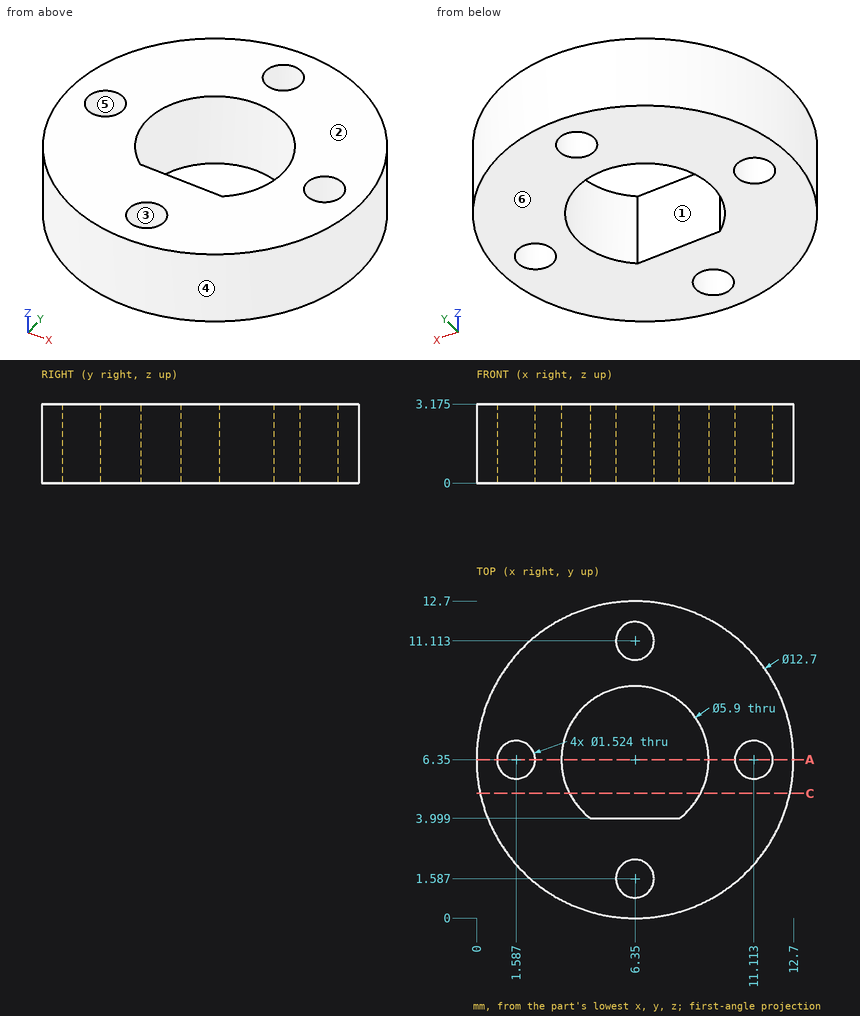
Print and shaded views of the part. All mm, measured from the part's lowest x, y and z. A direction names the side the tool comes from. Round coordinates to 2 decimals unless told otherwise and drop trailing zeros. Write each loop counter-clockwise with the first axis right and the second up, starting at its lowest first coordinate (ties: lowest second). Pieces come first, ordered by that corner, then holes. Notation, with made-up numbers: (33.25, 60) - (61.25, 60) arc R29 cw to (61.25, 92) - close; hole circle Ø1 at (26.25, 51). An arc over 180 degrees is marked (long way). Write each question's results on one line, items separated by ' | '. Start each with the question number.
Item 1: Drop flat-ended pins along their axis: P1, Ø1, axis at y = 5, z = 1, coming from the -X side; P2, Ø1.5, axis at y = 11, z = 0.5, coming from the -X side; P3, Ø1, axis at x = 1.5, z = 2.5, coming from the -Y side (1 decimal). Give the stop position or say it passes through.
Item 2: Mould opens along Y. For the marked faces 3, 4, 5 and 6 say: pulls with the +Y half, pulls with the -Y half, needs draft (parallel to the pull), parting line crosses it, or undercut.
Item 3: Saw through at A-A (y = 6.35). State how many separate pieces and enclosed holes the cut face has, and give its area (3 significant figures).
Item 4: Saw through at C-C (y = 5). Write the cut outline in (x, z) (1 decimal).
Item 5: Which spindle directions (+Z, -Z, +X, -X, +Y, -Y) get a long thin tool onto all of the face, cutting with end or side? Do the marked faces 1 and 2. Say none if no direction does.
Item 6: Wall check: L1, parallel to X at y = 7, z = 2.2 (1 decimal); L2, parallel to Y at x = 5, z = 2.2 (1 decimal); L3, parallel to X at y = 6.25, z = 1.1. Give the ranges that are in metal, low to high. Write a range as [from, to].
Results are:
1) P1: stops at x = 0.06 | P2: stops at x = 1.34 | P3: stops at y = 1.7
2) face 3: undercut | face 4: parting line crosses it | face 5: undercut | face 6: needs draft
3) separate pieces: 4 | enclosed holes: 0 | area: 11.9 mm²
4) outline: (0.1, 0) - (3.7, 0) - (3.7, 3.2) - (0.1, 3.2) - close; (9, 0) - (12.6, 0) - (12.6, 3.2) - (9, 3.2) - close
5) face 1: +Z, -Z | face 2: +Z, +X, -X, +Y, -Y
6) L1: x = [0, 1.2], [2, 3.5], [9.2, 10.7], [11.5, 12.7] | L2: y = [0.1, 4], [9, 12.6] | L3: x = [0, 0.83], [2.34, 3.4], [9.3, 10.36], [11.87, 12.7]
